```python
from build123d import *

# Parameters (mm, degrees)
F0_W     = 135
F0_H     = 65
F0_R     = 3.25
F0_R_2   = 4
F1_DEPTH = 10
F3_ANGLE = -180


with BuildPart() as f1:
    # F0 (on Top) → F1 (new body)
    with BuildSketch(Plane.XY):
        Rectangle(F0_W, F0_H)
        with Locations((-57.5, -22.5)):
            Circle(F0_R, mode=Mode.SUBTRACT)
        with Locations((57.5, -22.5)):
            Circle(F0_R, mode=Mode.SUBTRACT)
        with Locations((-20, 0)):
            Circle(F0_R_2, mode=Mode.SUBTRACT)
        with Locations((-57.5, 22.5)):
            Circle(F0_R, mode=Mode.SUBTRACT)
        with Locations((20, 0)):
            Circle(F0_R_2, mode=Mode.SUBTRACT)
        with Locations((57.5, 22.5)):
            Circle(F0_R, mode=Mode.SUBTRACT)
    extrude(amount=F1_DEPTH)

    # F2 (on face) → F3 (revolve)
    with BuildSketch(Plane.XY.offset(10)):
        Polygon((40, 0), (0, 0), (-40, 0), (-40, -95), (0, -95), (40, -95), align=None)
        Polygon((-40, -95), (-40, 0), (-45, 0), (-45, -100), (-40, -100), align=None)
        Polygon((45, 0), (40, 0), (40, -95), (40, -100), (45, -100), align=None)
    revolve(axis=Axis((-5.601771, 0, 10), (1, 0, 0)), revolution_arc=F3_ANGLE)


solid = f1.part
```
Input: part model. Units: mm. Frame: model coordinates. A direction names the side the tool comes from. Coordinates: 2 decimals unless noted, no trailing zeros. Write each loop counter-clockwise with the first axis right and the second up, starting at its lowest first coordinate (ties: lowest second). Pieces come first, ordered by that corner, then holes. Notation, with made-up numbers: (-21.75, -3.75) -> (36.25, -3.75) arc R25 cw to (36.25, 21.25) -> close; hole circle Ø4 at (-11.5, 37). An arc over 180 degrees is marked (long way). Write each question's results on one line, items separated by ' | '.
Item 1: Pin query (flat end, axial travel): pin 1 Ø6 at (x, y) = (57.5, 22.5) entering from +Z; pin 2 Ø20 at (x, y) = (-6, 65) entering from -Z; pin 3 Ø12 at (x, z) = (-46.5, 77.5) entering from -Y; pin 4 Ø8.5 at (x, y) = (-57.5, -22.5) entering from +Z. Return the tip coordinate at first contact, or that it passes through.
Conclusion:
pin 1: passes through | pin 2: stops at z = 10 | pin 3: stops at y = -78.7 | pin 4: stops at z = 10
Item 2: Set-up query: faces 1 (the flat face through (56, 0, 10)), 2 (the flat face through (-56, 0, 10)), 3 (the cylindrical face through (16.8, -2.4, 4.9)). Return all of +Z, -Z, +X, -X, +Y, -Y with unobstructed straight access to the full face (end or side cutting, diameter ignored); none if empty.
Conclusion:
face 1: +Z, +X, +Y, -Y | face 2: +Z, -X, +Y, -Y | face 3: -Z
Item 3: Section query D-D on z = 53. Return loops of the section in (x, y).
Conclusion:
outline: (-45, -90.28) -> (-40, -90.28) -> (-40, -84.71) -> (40, -84.71) -> (40, -90.28) -> (45, -90.28) -> (45, 90.28) -> (40, 90.28) -> (40, 84.71) -> (-40, 84.71) -> (-40, 90.28) -> (-45, 90.28) -> close
Item 4: Section query B-B on y = -22.5. Return loops of the section in (x, z), plus the area to 3 significant figures.
Conclusion:
outline: (-67.5, 0) -> (-60.75, 0) -> (-60.75, 10) -> (-67.5, 10) -> close; (-54.25, 0) -> (54.25, 0) -> (54.25, 10) -> (45, 10) -> (45, 107.44) -> (40, 107.44) -> (40, 102.3) -> (-40, 102.3) -> (-40, 107.44) -> (-45, 107.44) -> (-45, 10) -> (-54.25, 10) -> close; (60.75, 0) -> (67.5, 0) -> (67.5, 10) -> (60.75, 10) -> close | area: 9,580 mm^2
Item 5: Section query C-C on x = 20. Return loops of the section in (y, z).
Conclusion:
outline: (-95, 10) -> (-32.5, 10) -> (-32.5, 0) -> (-4, 0) -> (-4, 10) -> (4, 10) -> (4, 0) -> (32.5, 0) -> (32.5, 10) -> (95, 10) arc R95 ccw to start
Item 6: Material intervals for probe 1 along X at (y, z) = (22, 4); probe 2 along Y at (x, z) = (-57, 7); probe 3 along Y at (x, z) = (-20, 3.5), sorted ascending.
Conclusion:
probe 1: x = -67.5 to -60.71, -54.29 to 54.29, 60.71 to 67.5 | probe 2: y = -32.5 to -25.71, -19.29 to 19.29, 25.71 to 32.5 | probe 3: y = -32.5 to -4, 4 to 32.5
Item 7: Mould query, pull axis Y, two halves, no side actions, for faces 4 (the cylindrical face through (54.253, -22.357, 4.93)), 5 (the cylindrical face through (0.56, -2.089, 104.977)), 6 (the flat face through (-1, 0, 0)). Classes: +Y half, -Y half, draft (parallel to the pull), parting line (faces both ways), or undercut.
Conclusion:
face 4: undercut | face 5: parting line | face 6: draft
Item 8: Section query A-A on x = 57.5. Return loops of the section in (y, z).
Conclusion:
outline: (-32.5, 0) -> (-25.75, 0) -> (-25.75, 10) -> (-32.5, 10) -> close; (-19.25, 0) -> (19.25, 0) -> (19.25, 10) -> (-19.25, 10) -> close; (25.75, 0) -> (32.5, 0) -> (32.5, 10) -> (25.75, 10) -> close
